Print and shaded views of the part. All mm, measured from the part's lowest x, y and z. A direction names the side the tool comes from. Round coordinates to 2 decimals unless told otherwise and drop trailing zeros. Order: outer loops, then holes, each group sorted by start corner. A loop starts at its lowest first (then second) coordinate and runs counter-clockwise, first axis right, second up.
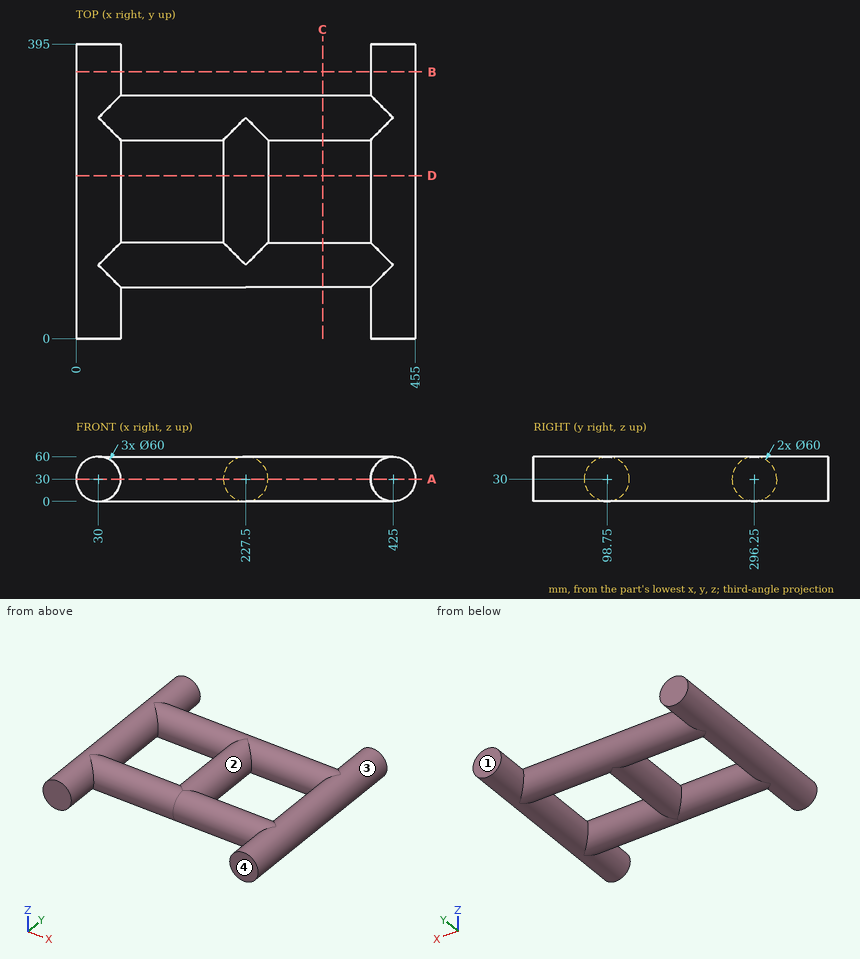
1. Cut at C-C, the plane x = 330.5. Write the cut outline in (y, z).
2. Cut at B-B, the plane y = 357.5. Write the cut outline in (x, z).
3. Mould opens along X. For the marked faces 3 and 4 say: released by +X, released by -X, zero draft, split by the parting line, or undercut.
4. Pin check, flat tips, straight feed: P1, Ø4, axis at y = 147, z = 27, coming from the +X side; P2, Ø8, axis at x = 130, z = 26, coming from the -Y side; P3, Ø6, axis at x = 109.5, z = 41, coming from the +Y side. Stop position of each tip, or through.
5. Drill centre lines: line 1 (X direction, y = 149.5, z = 8); line 2 (Y direction, x = 332, z = 28); line 3 (X direction, y = 259, z = 3.5). Where is each one in solid material? Low to high.
6. Tool access for the marked faces 1 and 2: list every direction of +Z, -Z, +X, -X, +Y, -Y with a clear straight run to the whole face (end or side of a thin tool).
7. Cut at D-D, the plane y = 218.5. Write the cut outline in (x, z).
8. Cut at A-A, the plane z = 30. Write the cut outline in (x, y).
Outcome:
1. outline: circle Ø60 at (98.75, 30); circle Ø60 at (296.25, 30)
2. outline: circle Ø60 at (30, 30); circle Ø60 at (425, 30)
3. face 3: undercut
3. face 4: zero draft
4. P1: stops at x = 454.98
4. P2: stops at y = 68.75
4. P3: stops at y = 325.16
5. line 1: x = 9.6 to 50.4, 207.1 to 247.9, 404.6 to 445.4
5. line 2: y = 68.82 to 128.68, 266.32 to 326.18
5. line 3: x = 15.94 to 44.06, 213.44 to 241.56, 410.94 to 439.06
6. face 1: +Z, -Z, +X, -X, +Y
6. face 2: none
7. outline: circle Ø60 at (30, 30); circle Ø60 at (227.5, 30); circle Ø60 at (425, 30)
8. outline: (0, 0) - (60, 0) - (60, 68.75) - (395, 68.75) - (395, 0) - (455, 0) - (455, 395) - (395, 395) - (395, 326.25) - (60, 326.25) - (60, 395) - (0, 395) - close; hole (60, 128.75) - (197.5, 128.75) - (197.5, 266.25) - (60, 266.25) - close; hole (257.5, 128.75) - (395, 128.75) - (395, 266.25) - (257.5, 266.25) - close
